from build123d import *

# Parameters (mm, degrees)
SKETCH2_R           = 4.7625
BOSS_EXTRUDE1_DEPTH = 3.175
LPATTERN1_COUNT     = 2
LPATTERN1_PITCH     = 6.35


with BuildPart() as part:
    # Sketch1 → Revolve1 (revolve)
    with BuildSketch(Plane.XY, mode=Mode.PRIVATE) as revolve1_sk:
        Polygon((0, 0), (1.9812, 0), (1.9812, 25.4), (3.175, 25.4), (3.175, 55.5625), (1.6637, 55.5625), (1.6637, 61.3283), (0, 61.3283), align=None)
    revolve(revolve1_sk.sketch.rotate(Axis((0, 0, 0), (0, 1, 0)), 90), axis=Axis((0, 0, 0), (0, 1, 0)))  # turned: the seam where the file's is

    # Sketch2 → Boss-Extrude1 (add)
    with BuildSketch(Plane.XZ.offset(-25.4)):
        with Locations(Location((0, 0, 0), (0, 0, 270))):  # turned: the seam where the file's is
            Circle(SKETCH2_R)
    extrude(amount=-BOSS_EXTRUDE1_DEPTH)

    # Sketch4 → Cut-Revolve1 (revolve, cut)
    with BuildSketch(Plane(origin=(0, 0, 0), x_dir=(0, 0, -1), z_dir=(1, 0, 0))):
        with BuildLine():
            Line((3.175, 39.1541), (3.175, 43.3959))
            ThreePointArc((3.175, 43.3959), (1.5875, 41.275), (3.175, 39.1541))
        make_face()
    cut_revolve1 = revolve(axis=Axis((0, 0, 0), (0, 1, 0)), mode=Mode.SUBTRACT)

    # LPattern1: Cut-Revolve1 ×2
    with Locations(*[(0, i * LPATTERN1_PITCH, 0) for i in range(1, LPATTERN1_COUNT)]):
        add(cut_revolve1, mode=Mode.SUBTRACT)


solid = part.part
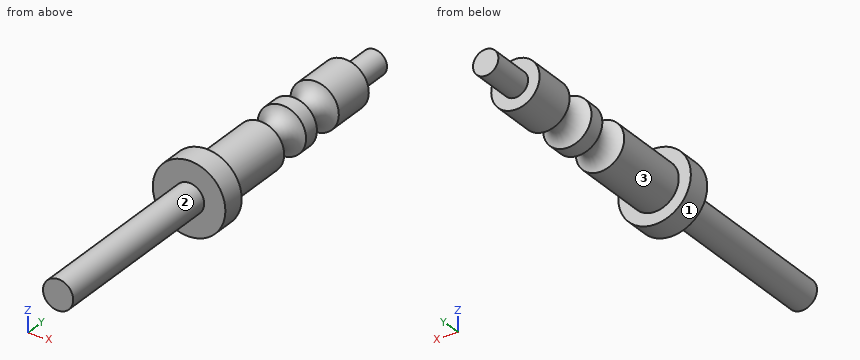
Can you work these out from the model? Positions are in its coordinate system, mm. Face numbers are marked on the shaded views. A direction names the side the tool comes from. Give positions to 0.01 mm unless a question says otherwise; leave off trailing zeros. Loops run counter-clockwise (first coordinate to the right, second up) from the corner with the lowest first, then second, coordinate; pieces in that order, holes last. Notation, with made-up numbers: (88.5, -21) -> (107.5, -21) arc R30 cw to (107.5, 4) -> close; hole circle Ø7 at (10, 65.5). An arc over 180 degrees is marked (long way). Write item = value, one per line.
1) Will these pins go through, and if not, where does the flat tip stop? pin 1 (3 mm diameter, centred on y = 39.5, z = -3.5, fed in from -X); pin 2 (5 mm diameter, centred on y = 32.5, z = -2, fed in from +X) (3 decimals); pin 3 (4 mm diameter, centred on x = 2, y = 22.5, fed in from -Z).
Check result:
pin_1 = -2.43
pin_2 = 3.175
pin_3 = -1.98
2) Suppose I cut it at B-B on x = 0. Write out the boundary of the cut face in (y, z) (1 decimal).
Check result:
outline = (0, -2) -> (25.4, -2) -> (25.4, -4.8) -> (28.6, -4.8) -> (28.6, -3.2) -> (39.2, -3.2) arc R2.2 cw to (43.4, -3.2) -> (45.5, -3.2) arc R2.2 cw to (49.7, -3.2) -> (55.6, -3.2) -> (55.6, -1.7) -> (61.3, -1.7) -> (61.3, 1.7) -> (55.6, 1.7) -> (55.6, 3.2) -> (49.7, 3.2) arc R2.2 cw to (45.5, 3.2) -> (43.4, 3.2) arc R2.2 cw to (39.2, 3.2) -> (28.6, 3.2) -> (28.6, 4.8) -> (25.4, 4.8) -> (25.4, 2) -> (0, 2) -> close
3) For the marked faces 1, 2 and 3, which set-ups out of +Z, -Z, +X, -X, +Y, -Y let a thin tool reach every point of the face, with its end or its side?
Check result:
face_1 = +Y, -Y
face_2 = -Y
face_3 = +Y
4) Suppose I cut it at C-C on y = 20. Write out the boundary of the cut face in (x, z), then the cut area to 3 significant figures.
Check result:
outline = circle Ø3.96 at (0, 0)
area = 12.3 mm2
5) I need wall thicknesses on L1, parallel to Y at x = 2.5, z = 0.5; L2, parallel to Y at x = -1.75, z = 2.25; L3, parallel to Y at x = 3.75, z = 1 (3 decimals). Which ranges of each line are inside material? Lowest first, please. Write a range as from..to.
Check result:
L1 = 25.4..39.45, 43.1..45.8, 49.45..55.56
L2 = 25.4..39.28, 43.27..45.63, 49.62..55.56
L3 = 25.4..28.575
6) Suppose I cut it at D-D on z = 4. Write out the boundary of the cut face in (x, y) (3 decimals), then the cut area to 3 significant figures.
Check result:
outline = (-2.585, 25.4) -> (2.585, 25.4) -> (2.585, 28.575) -> (-2.585, 28.575) -> close
area = 16.4 mm2
7) Suppose I cut it at A-A on z = 0. Write out the boundary of the cut face in (x, y) (1 decimal).
Check result:
outline = (-4.8, 25.4) -> (-2, 25.4) -> (-2, 0) -> (2, 0) -> (2, 25.4) -> (4.8, 25.4) -> (4.8, 28.6) -> (3.2, 28.6) -> (3.2, 39.2) arc R2.2 cw to (3.2, 43.4) -> (3.2, 45.5) arc R2.2 cw to (3.2, 49.7) -> (3.2, 55.6) -> (1.7, 55.6) -> (1.7, 61.3) -> (-1.7, 61.3) -> (-1.7, 55.6) -> (-3.2, 55.6) -> (-3.2, 49.7) arc R2.2 cw to (-3.2, 45.5) -> (-3.2, 43.4) arc R2.2 cw to (-3.2, 39.2) -> (-3.2, 28.6) -> (-4.8, 28.6) -> close
